Autodesk Inventor part; units mm, degrees
ref_plane "YZ Plane" through (0, 0, 0) normal (1, 0, 0) x (0, 1, 0)
ref_plane "XZ Plane" through (0, 0, 0) normal (0, 1, 0) x (-1, 0, 0)
ref_plane "XY Plane" through (0, 0, 0) normal (0, 0, 1) x (1, 0, 0)
sketch "Sketch1" plane through (0, 0, 0) normal (0, 1, 0) x (-1, 0, 0)
  line L0 (0, 0) -> (25.4, 0)
  line L1 (25.4, 0) -> (25.4, -25.4)
  line L2 (25.4, -25.4) -> (0, -25.4)
  line L3 (0, -25.4) -> (0, 0)
  dimension "d0" = 25.4
  dimension "d1" = 25.4
extrude "Extrusion1" add sketch "Sketch1" along normal blind 1.27
sketch "Sketch2" plane through (0, 0, 0) normal (0, -1, 0) x (1, 0, 0)
  line L0 (-6.6675, -6.6675) -> (-18.7325, -6.6675)
  line L1 (-18.7325, -6.6675) -> (-18.7325, -18.7325)
  line L2 (-18.7325, -18.7325) -> (-6.6675, -18.7325)
  line L3 (-6.6675, -18.7325) -> (-6.6675, -6.6675)
  line L4 (0, 0) -> (0, -25.4)
  line L5 (0, -25.4) -> (-25.4, -25.4)
  line L6 (-7.9375, -7.9375) -> (-17.4625, -7.9375)
  line L7 (-17.4625, -7.9375) -> (-17.4625, -17.4625)
  line L8 (-17.4625, -17.4625) -> (-7.9375, -17.4625)
  line L9 (-7.9375, -17.4625) -> (-7.9375, -7.9375)
  point P0 (-6.6675, -12.7)
  point P1 (0, -12.7)
  point P2 (-12.7, -18.7325)
  point P3 (-12.7, -25.4)
  dimension "d4" = 12.065
  dimension "d6" = 1.27
extrude "Extrusion2" add sketch "Sketch2" along normal blind 6.35
sketch "Sketch3" plane through (-18.7325, 0, -6.6675) normal (0, 0, 1) x (1, 0, 0)
  line L0 (3.175, -2.54) -> (8.89, -2.54)
  line L1 (8.89, -2.54) -> (8.89, -2.794)
  line L2 (8.89, -2.794) -> (3.175, -2.794)
  line L3 (3.175, -2.794) -> (3.175, -2.54)
  line L4 (12.065, -6.35) -> (0, -6.35)
  line L5 (-6.6675, 0) -> (18.7325, 0)
  line L6 (3.175, -0.889) -> (3.429, -0.889)
  line L7 (3.429, -0.889) -> (3.429, -2.794)
  line L8 (3.429, -2.794) -> (3.175, -2.794)
  line L9 (3.175, -2.794) -> (3.175, -0.889)
  line L10 (6.0325, -2.794) -> (6.0325, -2.54) construction
  line L11 (8.89, -0.889) -> (8.636, -0.889)
  line L12 (8.636, -0.889) -> (8.636, -2.794)
  line L13 (8.89, -2.794) -> (8.89, -0.889)
  point P0 (6.0325, -6.35)
  point P1 (8.636, -2.54)
  point P2 (3.429, -2.54)
  dimension "d9" = 0.254
  dimension "d10" = 5.715
  dimension "d11" = 2.54
  dimension "d14" = 0.254
  dimension "d15" = 1.905
extrude "Extrusion3" cut sketch "Sketch3" against normal through all
chamfer "Chamfer1" distance 0.508 angle 15 1 edges at (-12.7, -2.54, -6.6675) measured on face at (-13.6525, -5.1647, -6.6675)
sketch "Sketch4" plane through (-10.0965, -2.54, -7.9375) normal (1, 0, 0) x (0, 0, -1)
  line L0 (-1.27, 0.508) -> (-1.1339, 0)
  line L1 (-1.27, 0.508) -> (-1.27, 1.27)
  line L2 (-1.27, 0.508) -> (-1.4742, 1.27)
  line L3 (-1.4742, 1.27) -> (-1.27, 1.27)
  line L4 (-1.27, 1.651) -> (0, 1.651) construction
  line L5 (-1.27, 1.651) -> (-1.27, 1.27) construction
  line L6 (-1.27, 0.508) -> (-1.27, 1.651) construction
  point P0 (-7.9375, 2.54)
  dimension "d22" = 0.381
extrude "Extrusion4" add sketch "Sketch4" against normal up to surface (5.207 mm away)
ref_plane "Work Plane1" through (-18.7325, 0, -12.7) normal (0, 0, 1) x (1, 0, 0)
chamfer "Chamfer2" distance 0.508 angle 15 1 edges at (-12.7, -2.54, -18.7325) measured on face at (-11.7475, -5.1647, -18.7325)
mirror "Mirror2" about plane through (-18.7325, 0, -12.7) normal (0, 0, 1) of "Extrusion4"
sketch "Sketch5" plane through (0, 1.27, 0) normal (0, 1, 0) x (1, 0, 0)
  line L0 (0, 25.4) -> (-25.4, 25.4)
  line L1 (-25.4, 25.4) -> (-25.4, 0)
  line L2 (-25.4, 0) -> (0, 0)
  line L3 (0, 0) -> (0, 25.4)
  line L4 (-24.13, 1.27) -> (-24.13, 24.13)
  line L5 (-24.13, 24.13) -> (-1.27, 24.13)
  line L6 (-1.27, 24.13) -> (-1.27, 1.27)
  line L7 (-1.27, 1.27) -> (-24.13, 1.27)
  dimension "d26" = 1.27
extrude "Extrusion5" cut sketch "Sketch5" against normal blind 0.254 contours L4 L5 L6 L7
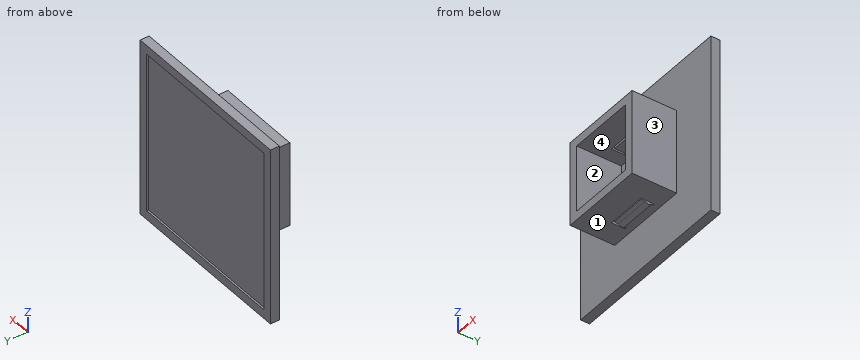
The listing builds one solid part. Answer for the finished solid, in the listing's coordinates (mm). Face numbers are marked on the shaded views. Round coordinates to 2 decimals unless told otherwise and drop trailing zeros. Loops run counter-clockwise (first coordinate to the right, second up) from the corner with the lowest first, then second, coordinate; pieces in that order, holes last. Notation, with made-up numbers: (55.25, 5.5) - (67.25, 5.5) arc R28 ccw to (67.25, 27.5) - close; hole circle Ø7 at (67, 39.5). An arc over 180 degrees is marked (long way). Return JSON: item names as keys, results as strings. Group by question number.
1. Consider probe 1 along Z at (x, y) = (-9.25, -3.5); probe 2 along Y at (x, z) = (-23.25, -20). Determine where each line is inside the solid, lowest interval first.
2. The mould has two halves that part along Z. Classify the marked faces 1, 2, 3 and 4: pulls with the +Z half, pulls with the -Z half, needs draft (parallel to the pull), parting line crosses it, or undercut.
3. The part is cut by section B-B on z = -13.25. Determine the outline of the cut face in (x, y).
4. Each of these flat-tipped pins is pushed along its axis until it touches: P1, Ø2, axis at x = -16.5, y = -5, coming from the -Z side; P2, Ø1.5, axis at y = -1, z = -10, coming from the -X side; P3, Ø1.5, axis at x = -4, z = -13, coming from the -Y side; P4, Ø11.5, axis at x = -18.5, z = -14, coming from the +Y side. Where does it stop, or does it pass through?
5. The part is cut by section A-A on x = -16. Determine the outline of the cut face in (y, z), then the cut area to 3 significant figures.
6. The part is cut by section D-D on z = -5. Determine the outline of the cut face in (x, y), then the cut area to 3 significant figures.
7. The part is cut by section C-C on y = -5. Determine the outline of the cut face in (x, z).
Resolved:
{
 "1": {"probe 1": "z = -18.73 to -17.46, -7.94 to -6.67", "probe 2": "y = 0 to 1.02"},
 "2": {"face 1": "pulls with the -Z half", "face 2": "undercut", "face 3": "needs draft", "face 4": "undercut"},
 "3": {"outline": "(-25.4, 0) - (-18.73, 0) - (-18.73, -6.35) - (-17.46, -6.35) - (-17.46, 0) - (-7.94, 0) - (-7.94, -6.35) - (-6.67, -6.35) - (-6.67, 0) - (0, 0) - (0, 1.27) - (-1.27, 1.27) - (-1.27, 1.02) - (-24.13, 1.02) - (-24.13, 1.27) - (-25.4, 1.27) - close"},
 "4": {"P1": "stops at z = -18.73", "P2": "stops at x = -18.73", "P3": "stops at y = 0", "P4": "stops at y = 1.27"},
 "5": {"outline": "(-6.35, -18.73) - (0, -18.73) - (0, -25.4) - (1.27, -25.4) - (1.27, -24.13) - (1.02, -24.13) - (1.02, -1.27) - (1.27, -1.27) - (1.27, 0) - (0, 0) - (0, -6.67) - (-6.35, -6.67) - (-6.35, -7.94) - (0, -7.94) - (0, -17.46) - (-6.35, -17.46) - close", "area": "42.6 mm²"},
 "6": {"outline": "(-25.4, 0) - (0, 0) - (0, 1.27) - (-1.27, 1.27) - (-1.27, 1.02) - (-24.13, 1.02) - (-24.13, 1.27) - (-25.4, 1.27) - close", "area": "26.5 mm²"},
 "7": {"outline": "(-18.73, -18.73) - (-6.67, -18.73) - (-6.67, -6.67) - (-18.73, -6.67) - close; hole (-17.46, -17.46) - (-7.94, -17.46) - (-7.94, -7.94) - (-17.46, -7.94) - close"}
}
